Job drawing, mm, ordinate dimensions from the low corner. One solid piece. A direction names the side the tool comes from. Round coordinates to 2 decimals unless told otherwise and drop trailing zeros. Loops run counter-clockwise (first coordinate to the right, second up) from the corner with the lowest first, then second, coordinate; pieces in that order, holes last. Notation, with made-up numbers: M 14,18 L 65,18 A13 cw 65,38 Z; hole C 28,-36.75 d9. An arc over 180 degrees is marked long. Write each question's results on one line, items separated by ' | '. Start each with the question number.
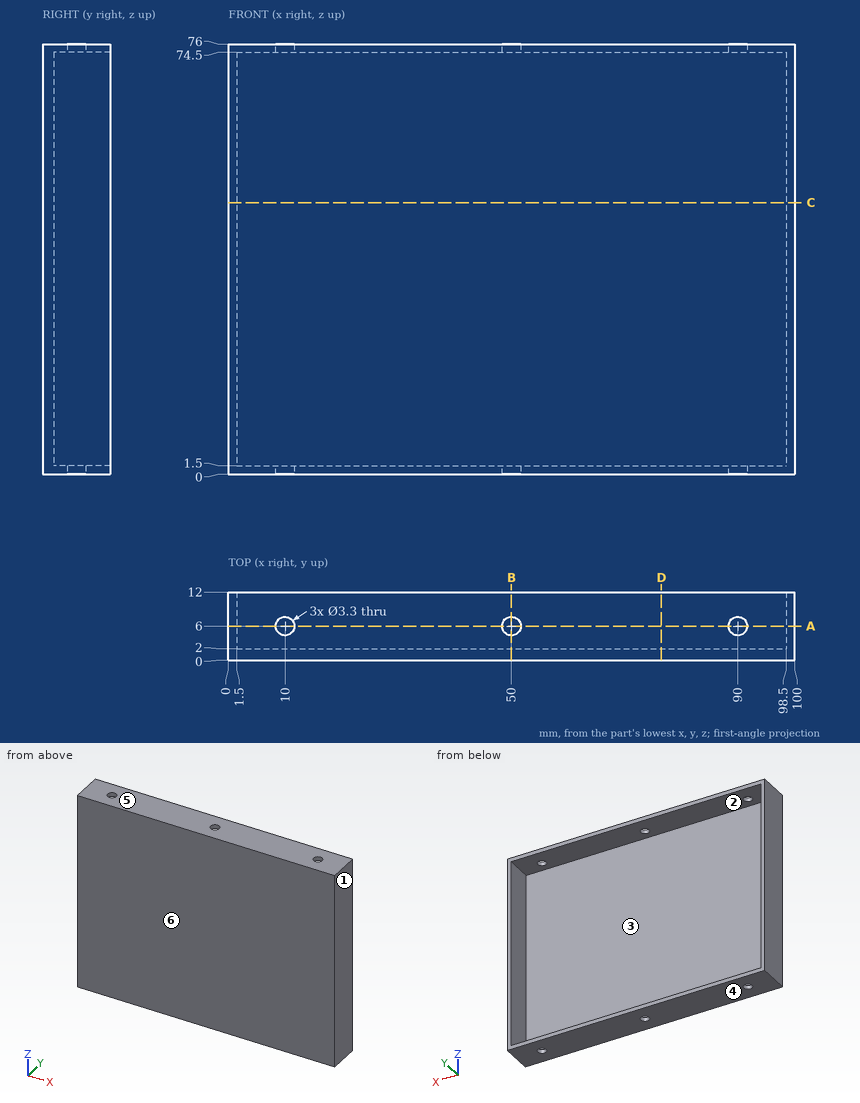
Item 1: Drop flat-ended pins along their axis: pin 1 (3 mm diameter, centred on x = 10, y = 6, fed in from -Z); pin 2 (3 mm diameter, centred on x = 56, z = 31, fed in from +Y). Give the stop position or say it passes through.
Item 2: Saw through at B-B, the plane x = 50. Give the cut face in (y, z), then the cut area to 3 significant figures.
Item 3: Saw through at A-A, the plane y = 6. State how many separate pieces and enclosed holes the cut face has, then the cut area to 3 significant figures.
Item 4: Saw through at D-D, the plane x = 76.5. Give the cut face in (y, z).
Item 5: Drill centre lines: line 1 along Y through (x, z) = (10, 75); line 2 along Z through (x, y) = (15, 6); line 3 along X through (y, z) = (9.5, 64.5). Where is each one in solid material? Low to high. Write a range as [from, to].
Item 6: Mould opens along Z. For the marked faces 3, 4, 5 and 6 say: released by +Z, released by -Z, zero draft, split by the parting line, or undercut.
Item 7: Saw through at C-C, the plane z = 48. Give the cut face in (x, y).
Item 8: Tool access for the marked faces 1 and 2: list every direction of +Z, -Z, +X, -X, +Y, -Y with a clear straight run to the whole face (end or side of a thin tool).
Working result:
1) pin 1: passes through | pin 2: stops at y = 2
2) outline: M 0,0 L 4.35,0 L 4.35,1.5 L 2,1.5 L 2,74.5 L 4.35,74.5 L 4.35,76 L 0,76 Z; M 7.65,0 L 12,0 L 12,1.5 L 7.65,1.5 Z; M 7.65,74.5 L 12,74.5 L 12,76 L 7.65,76 Z | area: 172 mm²
3) separate pieces: 6 | enclosed holes: 0 | area: 489 mm²
4) outline: M 0,0 L 12,0 L 12,1.5 L 2,1.5 L 2,74.5 L 12,74.5 L 12,76 L 0,76 Z
5) line 1: y = [0, 4.35], [7.65, 12] | line 2: z = [0, 1.5], [74.5, 76] | line 3: x = [0, 1.5], [98.5, 100]
6) face 3: undercut | face 4: released by -Z | face 5: released by +Z | face 6: zero draft
7) outline: M 0,0 L 100,0 L 100,12 L 98.5,12 L 98.5,2 L 1.5,2 L 1.5,12 L 0,12 Z
8) face 1: +Z, -Z, +X, +Y, -Y | face 2: +Y
